from build123d import *

# Parameters (mm, degrees)
SKETCH1_W           = 28.89
SKETCH1_H           = 18.5
BOSS_EXTRUDE1_DEPTH = 7.22
SKETCH2_R           = 6
BOSS_EXTRUDE2_DEPTH = 18.75
BOSS_EXTRUDE3_DEPTH = 2.9
SKETCH4_W           = 1.6
SKETCH4_H           = 10.5
BOSS_EXTRUDE4_DEPTH = 3.1


with BuildPart() as part:
    # Sketch1 → Boss-Extrude1 (new, symmetric)
    with BuildSketch(Plane.XY):
        Rectangle(SKETCH1_W, SKETCH1_H)
    extrude(amount=BOSS_EXTRUDE1_DEPTH, both=True)

    # Sketch2 → Boss-Extrude2 (add)
    with BuildSketch(Plane(origin=(0, 0, 0), x_dir=(1, 0, 0), z_dir=(0, 1, 0))):
        with Locations(Location((0, 0, 0), (0, 0, 90))):
            Circle(SKETCH2_R)
    extrude(amount=BOSS_EXTRUDE2_DEPTH)

    # Sketch3 → Boss-Extrude3 (add, symmetric)
    with BuildSketch(Plane.XY):
        Polygon((-0.986, 17.391), (0.986, 18.109), (-4.644, 35.199), (-6.636315055, 34.542666837), align=None)
    extrude(amount=BOSS_EXTRUDE3_DEPTH, both=True)

    # Sketch4 → Boss-Extrude4 (add, symmetric)
    with BuildSketch(Plane.XY):
        with Locations((-8, -14.5)):
            Rectangle(SKETCH4_W, SKETCH4_H)
        with Locations((8, -14.5)):
            Rectangle(SKETCH4_W, SKETCH4_H)
    extrude(amount=BOSS_EXTRUDE4_DEPTH, both=True)


solid = part.part
Read the model definition and answer for the solid it produces. Units are mm, in the model's axes. A direction names the side the tool comes from. Coordinates: 2 decimals unless noted, no trailing zeros. Write each loop counter-clockwise with the first axis right and the second up, starting at its lowest first coordinate (ties: lowest second). Pieces come first, ordered by that corner, then holes. Notation, with made-up numbers: M 78.5,71 L 92.5,71 A24 ccw 92.5,85 Z; hole C -14,-7.5 d11. An arc over 180 degrees is marked long. Use a Markdown table: item, result.
Q1. Each of these flat-tipped pins is pushed along its axis until it touches: pin 1 Ø2 at (x, y) = (-4, 23.5) entering from +Z; pin 2 Ø1 at (x, z) = (7.5, 5) entering from -Y; pin 3 Ø6 at (x, y) = (-4.5, 24.5) entering from -Z. Where does it stop, or does it pass through?
Answer block:
| item | result |
|---|---|
| pin 1 | stops at z = 2.9 |
| pin 2 | stops at y = -9.25 |
| pin 3 | stops at z = -2.9 |
Q2. Determine the mould class of faces 1 (the face through (-7.2, -15, 0)), 2 (the face through (-4.071, 26.757, 0.041)), 3 (the face through (-1.897, 26.859, 0.041)), 4 (the face through (1, 18.75, 0)) for opening direction Y: released by +Y, released by -Y, zero draft, split by the parting line, or undercut.
Answer block:
| item | result |
|---|---|
| face 1 | zero draft |
| face 2 | undercut |
| face 3 | released by +Y |
| face 4 | undercut |
Q3. The part is cut by section B-B, the plane x = 8.25. Write down the section's boundary in (y, z), then the cut area to 3 significant figures.
Answer block:
| item | result |
|---|---|
| outline | M -19.75,-3.1 L -9.25,-3.1 L -9.25,-7.22 L 9.25,-7.22 L 9.25,7.22 L -9.25,7.22 L -9.25,3.1 L -19.75,3.1 Z |
| area | 332 mm2 |
Q4. The part is cut by section D-D, the plane y = 30.5. Write down the section's boundary in (x, z).
Answer block:
| item | result |
|---|---|
| outline | M -5.3,-2.9 L -3.1,-2.9 L -3.1,2.9 L -5.3,2.9 Z |
Q5. Straight lines are drawn through the part: L1, parallel to X at y = -12, z = 0.5; L2, parallel to Y at x = -7.5, z = 3; L3, parallel to Y at x = 9.5, z = -6. For each, find the intervals that lie inside material, in ascending order. Write a range as [from, to].
Answer block:
| item | result |
|---|---|
| L1 | x = [-8.8, -7.2], [7.2, 8.8] |
| L2 | y = [-19.75, 9.25] |
| L3 | y = [-9.25, 9.25] |
Q6. Which of the six approach directions +Z, -Z, +X, -X, +Y, -Y give full straight-line access (tool end or side, diameter ignored) to faces 5 (the face through (8, -14, -3.1)), 6 (the face through (8, -14, 3.1)), 7 (the face through (7.2, -15, 0)), 8 (the face through (8.8, -15, 0))?
Answer block:
| item | result |
|---|---|
| face 5 | -Z, +X, -X, -Y |
| face 6 | +Z, +X, -X, -Y |
| face 7 | +Z, -Z, -Y |
| face 8 | +Z, -Z, +X, -Y |
Q7. The part is cut by section A-A, the plane y = -13. Write down the section's boundary in (x, z), then the cut area to 3 significant figures.
Answer block:
| item | result |
|---|---|
| outline | M -8.8,-3.1 L -7.2,-3.1 L -7.2,3.1 L -8.8,3.1 Z; M 7.2,-3.1 L 8.8,-3.1 L 8.8,3.1 L 7.2,3.1 Z |
| area | 19.8 mm2 |
Q8. The part is cut by section C-C, the plane z = 0. Write down the section's boundary in (x, y) (3 decimals), then the cut area to 3 significant figures.
Answer block:
| item | result |
|---|---|
| outline | M -14.445,-9.25 L -8.8,-9.25 L -8.8,-19.75 L -7.2,-19.75 L -7.2,-9.25 L 7.2,-9.25 L 7.2,-19.75 L 8.8,-19.75 L 8.8,-9.25 L 14.445,-9.25 L 14.445,9.25 L 6,9.25 L 6,18.75 L 0.775,18.75 L -4.644,35.199 L -6.636,34.543 L -1.434,18.75 L -6,18.75 L -6,9.25 L -14.445,9.25 Z |
| area | 718 mm2 |
